Input: part model. Units: mm. Frame: model coordinates. Coordinates: 2 decimals unless noted, no trailing zeros. Loops run counter-clockwise (first coordinate to the right, second up) from the corner with the lowest first, then second, coordinate; pieces in that order, holes last.
(1) Contact query for flat-ended pins moving along their axis: P1, Ø7, axis at x = 0, y = 0, coming from the -Z side; P2, Ø1, axis at y = 7.5, z = 2, coming from the -X side. Output: stop coordinate, or through.
(2) Line query: L1, parallel to X at y = -2.25, z = 0.7; L2, parallel to Y at x = -1.75, z = 1.65; L3, parallel to Y at x = 2.25, z = 1.45. Output: solid intervals per line, ascending.
(3) Section B-B, the plane z = 2.45. Return loops of the section in (x, y).
(4) Section A-A, the plane x = -2.25. Return loops of the section in (y, z).
(5) Section C-C, the plane x = 8. Return loops of the section in (y, z), then the cut area to 3 significant figures.
(6) Mould query, pull axis Y, two halves, no side actions, for faces 1 (the face through (11.78, 8.41, 1.48)), 2 (the face through (-7.24, 11.19, 1.48)), 3 (the face through (1.44, 2.26, 1.48)). Classes: released by +Y, released by -Y, zero draft, split by the parting line, or undercut.
```python
from build123d import *

# Parameters (mm, degrees)
F1_R     = 2.679687
F2_DEPTH = 3


with BuildPart() as f2:
    # F1 (on Top) → F2 (new body)
    with BuildSketch(Plane.XY):
        with BuildLine():
            Line((1.104634, 20.705122), (-6.082774, 13.244711))
            ThreePointArc((-6.082774, 13.244711), (-7.2458, 11.159807), (-7.229049, 8.772513))
            Line((-7.229049, 8.772513), (-4.516401, -1.225397))
            ThreePointArc((-4.516401, -1.225397), (-3.324232, -3.293775), (-1.266915, -4.504931))
            Line((-1.266915, -4.504931), (8.705599, -7.309485))
            ThreePointArc((8.705599, -7.309485), (13.266291, -6.128786), (14.488918, -1.579154))
            Line((14.488918, -1.579154), (8.991166, 18.683715))
            ThreePointArc((8.991166, 18.683715), (5.63666, 21.991473), (1.104634, 20.705122))
        make_face()
        Circle(F1_R, mode=Mode.SUBTRACT)
        with Locations((9.972518, -2.804555)):
            Circle(F1_R, mode=Mode.SUBTRACT)
        with Locations((-2.712648, 9.997909)):
            Circle(F1_R, mode=Mode.SUBTRACT)
        with Locations((4.474763, 17.458323)):
            Circle(F1_R, mode=Mode.SUBTRACT)
    extrude(amount=F2_DEPTH)


solid = f2.part
```
Report:
1. P1: stops at z = 0
1. P2: stops at x = -7.02
2. L1: x = -4.1 to -1.46, 1.46 to 7.35, 12.59 to 14.62
2. L2: y = -4.34 to -2.03, 2.03 to 7.5, 12.5 to 17.74
2. L3: y = -5.49 to -1.46, 1.46 to 15.96, 18.95 to 21.58
3. outline: (-7.23, 8.77) - (-4.52, -1.23) arc R4.68 ccw to (-1.27, -4.5) - (8.71, -7.31) arc R4.68 ccw to (14.49, -1.58) - (8.99, 18.68) arc R4.68 ccw to (1.1, 20.71) - (-6.08, 13.24) arc R4.68 ccw to start; hole circle Ø5.36 at (-2.71, 10); hole circle Ø5.36 at (0, 0); hole circle Ø5.36 at (4.47, 17.46); hole circle Ø5.36 at (9.97, -2.8)
4. outline: (-4.1, 0) - (-1.46, 0) - (-1.46, 3) - (-4.1, 3) - close; (1.46, 0) - (7.36, 0) - (7.36, 3) - (1.46, 3) - close; (12.64, 0) - (17.22, 0) - (17.22, 3) - (12.64, 3) - close
5. outline: (-7.11, 0) - (-4.62, 0) - (-4.62, 3) - (-7.11, 3) - close; (-0.99, 0) - (20.54, 0) - (20.54, 3) - (-0.99, 3) - close
5. area: 72.1 mm2
6. face 1: released by +Y
6. face 2: split by the parting line
6. face 3: undercut
